The drawing under review shows one solid part. Ordinate dimensions are in mm from its lowest x, y, z. A direction names the side the tool comes from. Give positions to 0.01 mm unless a question says otherwise; leave off trailing zeros. Loops run counter-clockwise (first coordinate to the right, second up) from the corner with the lowest first, then second, coordinate; pieces in that order, holes last. Notation, with made-up numbers: (-8.75, -5.75) - (12.25, -5.75) arc R37 ccw to (12.25, 30.25) - close; hole circle Ø4 at (87.25, 74.25). An arc over 180 degrees is marked (long way). One line per item, written item: value. Start each with the question number.
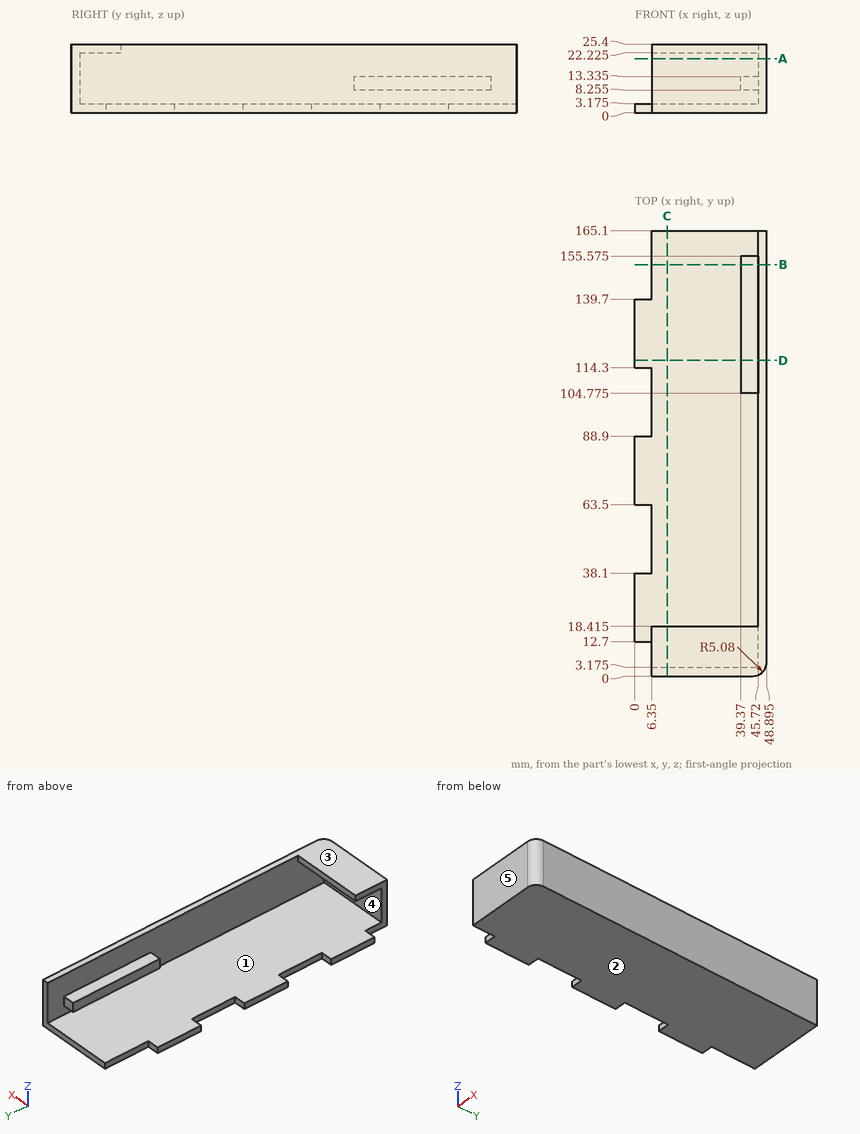
(1) Take a section at A-A on z = 20. State the section outline as (x, y) points (3 decimals).
(2) Draft analysis for pull direction Z (two halves, no side actions). For the marked faces 3, 4 and 5, state which applies: pulls with the +Z half, pulls with the -Z half, needs draft (parallel to the pull), parting line crosses it, or undercut.
(3) Take a section at B-B on y = 152.5. State the section outline as (x, z) points (3 decimals), and give its area (3 significant figures).
(4) Take a section at D-D on y = 117. State the section outline as (x, z) points (3 decimals), and give its area (3 significant figures).
(5) Machinability: for the marked faces 1 and 2, which of the approach directions +Z, -Z, +X, -X, +Y, -Y give a long, thin tool a straight path to every point of the face, cutting with its end or side? Answer none if there is none.
(6) To check wall thickness, follow L1, parallel to Y at x = 6.5, z = 16.75 (3 decimals); L2, parallel to X at y = 155, z = 24.5 (3 decimals). State the ranges of each line that lie inside material, in increasing order. Write a range as from..to.
(7) Take a section at C-C on x = 12. State the section outline as (y, z) points (3 decimals).
(8) For pin 1 Ø6 at (y, z) = (99, 19.5) entering from -X; pin 2 Ø8 at (x, y) = (35, 126) entering from +Z (3 decimals); pin 3 Ø1.6 at (y, z) = (101, 2) entering from -X, all flat-tipped, find the tip position at first contact; note any pin that passes through.
Here are the results:
1. outline: (6.35, 0) - (43.815, 0) arc R5.08 ccw to (48.895, 5.08) - (48.895, 165.1) - (45.72, 165.1) - (45.72, 3.175) - (6.35, 3.175) - close
2. face 3: pulls with the +Z half
2. face 4: undercut
2. face 5: needs draft
3. outline: (6.35, 0) - (48.895, 0) - (48.895, 25.4) - (45.72, 25.4) - (45.72, 13.335) - (39.37, 13.335) - (39.37, 8.255) - (45.72, 8.255) - (45.72, 3.175) - (6.35, 3.175) - close
3. area: 238 mm²
4. outline: (0, 0) - (48.895, 0) - (48.895, 25.4) - (45.72, 25.4) - (45.72, 13.335) - (39.37, 13.335) - (39.37, 8.255) - (45.72, 8.255) - (45.72, 3.175) - (0, 3.175) - close
4. area: 258 mm²
5. face 1: -X, +Y
5. face 2: -Z, +X, -X, +Y, -Y
6. L1: 0..3.175
6. L2: 45.72..48.895
7. outline: (0, 0) - (165.1, 0) - (165.1, 3.175) - (3.175, 3.175) - (3.175, 22.225) - (18.415, 22.225) - (18.415, 25.4) - (0, 25.4) - close
8. pin 1: x = 45.72
8. pin 2: z = 3.175
8. pin 3: x = 6.35
